```python
from build123d import *

# Parameters (mm, degrees)
PAD_DEPTH       = 10
SKETCH001_R     = 1.5
POCKET_DEPTH    = 10.001
FILLET_R        = 3
POCKET001_DEPTH = 10.001
FILLET001_R     = 2


with BuildPart() as part:
    # Sketch → Pad (new body)
    with BuildSketch(Plane.XZ):
        Polygon((52.5, 0), (52.5, 24.328), (67.5019, 18.2611), (92.4761, 18.2611), (107.478, 24.328), (107.478, 0), align=None)
    extrude(amount=PAD_DEPTH)

    # Sketch001 → Pocket (cut, through all)
    with BuildSketch(Plane(origin=(0, 0, 0), x_dir=(1, 0, 0), z_dir=(0, 1, 0))):
        with Locations((100.483, -12.3298)):
            Circle(SKETCH001_R)
        with Locations((59.458744, -12.3298)):
            Circle(SKETCH001_R)
    extrude(amount=-POCKET_DEPTH, mode=Mode.SUBTRACT)

    # Fillet
    fillet_edges = [part.edges().sort_by_distance(p)[0] for p in [
        (52.5, -5, 24.328),
        (107.478, -5, 24.328),
    ]]
    fillet(fillet_edges, radius=FILLET_R)

    # Sketch002 → Pocket001 (cut, through all)
    with BuildSketch(Plane.XZ.offset(10)):
        Polygon((56.5, 0), (56.5, 9.5), (63, 9.5), (63, 14.5), (97, 14.5), (97, 9.5), (103.5, 9.5), (103.5, 0), align=None)
    extrude(amount=-POCKET001_DEPTH, mode=Mode.SUBTRACT)

    # Fillet001
    fillet001_edges = [part.edges().sort_by_distance(p)[0] for p in [
        (63, -5, 9.5),
        (97, -5, 9.5),
    ]]
    fillet(fillet001_edges, radius=FILLET001_R)


solid = part.part
```
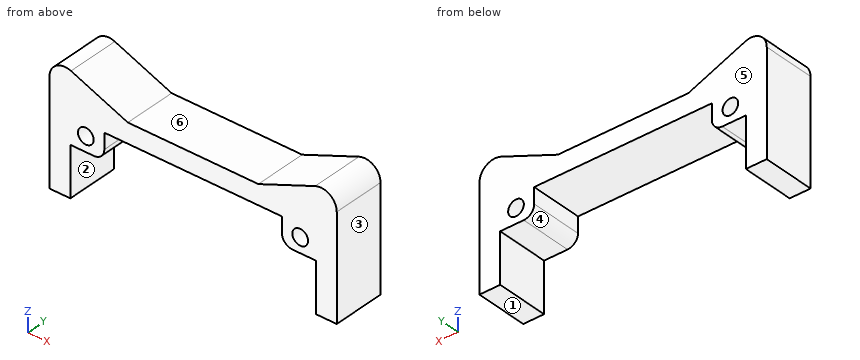
Check sheet for the modelled part. Datum: model origin and axes. Units: mm. Face numbers are marked on the shaded views. A direction names the side the tool comes from. Coordinates: 2 decimals unless noted, no trailing zeros. Write each loop counter-clockwise with the first axis right and the second up, starting at its lowest first coordinate (ties: lowest second). Pieces come first, ordered by that corner, then holes. Notation, with made-up numbers: (-12.75, -22) - (25.25, -22) arc R16 cw to (25.25, -14) - close; hole circle Ø7 at (65, 84.5). An arc over 180 degrees is marked (long way). One line per question, with ' | ' between items.
Item 1: Sectioned sample at B-B on z = 13. Record the boundary of the cut face in (x, y).
Determined:
outline: (52.5, -10) - (58.12, -10) - (58.12, 0) - (52.5, 0) - close; (60.8, -10) - (63, -10) - (63, 0) - (60.8, 0) - close; (97, -10) - (99.14, -10) - (99.14, 0) - (97, 0) - close; (101.82, -10) - (107.48, -10) - (107.48, 0) - (101.82, 0) - close
Item 2: Gauge pin test, flat ends, axial feed: P1, Ø3.5, axis at x = 59, y = -4.5, coming from the -Z side; P2, Ø3, axis at x = 85.5, y = -3, coming from the -Z side; P3, Ø5, axis at x = 82, z = 13, coming from the -Y side. Record the tip position at first contact, or that the pin passes through.
Determined:
P1: stops at z = 9.5 | P2: stops at z = 14.5 | P3: stops at y = -10
Item 3: Mould release check, pull along X, two halves, no side actions. Record for the marked faces 1, 2 and 3: pulls with the +X half, pulls with the -X half, needs draft (parallel to the pull), parting line crosses it, or undercut.
Determined:
face 1: needs draft | face 2: undercut | face 3: pulls with the +X half
Item 4: Sectioned sample at A-A on z = 8.25. Record the boundary of the cut face in (x, y).
Determined:
outline: (52.5, -10) - (56.5, -10) - (56.5, 0) - (52.5, 0) - close; (103.5, -10) - (107.48, -10) - (107.48, 0) - (103.5, 0) - close
Item 5: Sectioned sample at D-D on x = 84.5. Record the boundary of the cut face in (y, z).
Determined:
outline: (-10, 14.5) - (0, 14.5) - (0, 18.26) - (-10, 18.26) - close
Item 6: Access from +Z, -Z, +X, -X, +Y, -Y to the whole of each face (thin tool, end or side, straight path). Record for the marked faces 4, 5 and 6.
Determined:
face 4: -Z, +Y, -Y | face 5: +Z, -Z, +X, -X, +Y | face 6: +Z, +Y, -Y
Item 7: Thickness scan on line 1 (X direction, y = -4.5, z = 7.75); line 2 (X direction, y = -8, z = 12); line 3 (Z direction, x = 82.5, y = -4). Record the ranges inside material, lowest first. Write a range as [from, to].
Determined:
line 1: x = [52.5, 56.5], [103.5, 107.48] | line 2: x = [52.5, 58], [60.92, 63], [97, 99.02], [101.95, 107.48] | line 3: z = [14.5, 18.26]
Item 8: Sectioned sample at C-C on y = -7.75. Record the boundary of the cut face in (x, z), plus the area to 3 significant figures.
Determined:
outline: (52.5, 0) - (56.5, 0) - (56.5, 9.5) - (61, 9.5) arc R2 ccw to (63, 11.5) - (63, 14.5) - (97, 14.5) - (97, 11.5) arc R2 ccw to (99, 9.5) - (103.5, 9.5) - (103.5, 0) - (107.48, 0) - (107.48, 19.88) arc R3 ccw to (103.35, 22.66) - (92.48, 18.26) - (67.5, 18.26) - (56.62, 22.66) arc R3 ccw to (52.5, 19.88) - close; hole circle Ø3 at (59.46, 12.33); hole circle Ø3 at (100.48, 12.33) | area: 454 mm2
